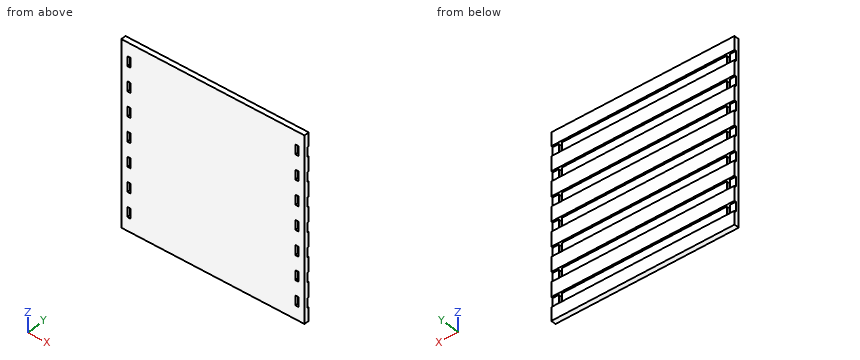
from build123d import *

# Parameters (mm, degrees)
SKETCH1_W           = 190.5
SKETCH1_H           = 190.5
BOSS_EXTRUDE1_DEPTH = 5.159375
SKETCH2_W           = 190.5
SKETCH2_H           = 10.16
CUT_EXTRUDE1_DEPTH  = 1.778
SKETCH3_W           = 3.175
SKETCH3_H           = 10.16
CUT_EXTRUDE3_DEPTH  = 4.381375
LPATTERN1_COUNT     = 7
LPATTERN1_PITCH     = 25.4


with BuildPart() as part:
    # Sketch1 → Boss-Extrude1 (new body)
    with BuildSketch(Plane(origin=(0, 0, 0), x_dir=(1, 0, 0), z_dir=(0, 1, 0))):
        Rectangle(SKETCH1_W, SKETCH1_H)
    extrude(amount=BOSS_EXTRUDE1_DEPTH)

    # Sketch2 → Cut-Extrude1 (cut)
    with BuildSketch(Plane(origin=(0, 5.159375, 0), x_dir=(1, 0, 0), z_dir=(0, 1, 0))):
        with Locations((0, 76.2)):
            Rectangle(SKETCH2_W, SKETCH2_H)
        with Locations((0, 50.8)):
            Rectangle(SKETCH2_W, SKETCH2_H)
        with Locations((0, 25.4)):
            Rectangle(SKETCH2_W, SKETCH2_H)
        Rectangle(SKETCH2_W, SKETCH2_H)
        with Locations((0, -25.4)):
            Rectangle(SKETCH2_W, SKETCH2_H)
        with Locations((0, -50.8)):
            Rectangle(SKETCH2_W, SKETCH2_H)
        with Locations((0, -76.2)):
            Rectangle(SKETCH2_W, SKETCH2_H)
    extrude(amount=-CUT_EXTRUDE1_DEPTH, mode=Mode.SUBTRACT)

    # Sketch3 → Cut-Extrude3 (cut, through all)
    with BuildSketch(Plane(origin=(0, 3.381375, 0), x_dir=(1, 0, 0), z_dir=(0, 1, 0))):
        with Locations((-87.3125, 76.2)):
            Rectangle(SKETCH3_W, SKETCH3_H)
        with Locations((87.3125, 76.2)):
            Rectangle(SKETCH3_W, SKETCH3_H)
    cut_extrude3 = extrude(amount=-CUT_EXTRUDE3_DEPTH, mode=Mode.SUBTRACT)

    # LPattern1: Cut-Extrude3 ×7
    with Locations(*[(0, 0, i * LPATTERN1_PITCH) for i in range(1, LPATTERN1_COUNT)]):
        add(cut_extrude3, mode=Mode.SUBTRACT)


solid = part.part
Input: part model. Units: mm. Frame: model coordinates. Give positions to 0.01 mm unless a question says otherwise; leave off trailing zeros. Order: outer loops, then holes, each group sorted by start corner. A loop starts at its lowest first (then second) coordinate and runs counter-clockwise, first axis right, second up.
Q1. Section B-B on y = 4.35. State how many separate pieces and enclosed holes the cut face has, and give its area (3 significant figures).
Checked values:
separate pieces: 8
enclosed holes: 0
area: 22,700 mm2
Q2. Contact query for a flat-ended pin moving along its axis: pin 1 Ø3 at (x, z) = (93, -48.5) entering from +Y. Output: stop coordinate, or through.
Checked values:
pin 1: stops at y = 3.38
Q3. Section A-A on z = -1. Output: boundary loops of the cut face in (x, y) (3 decimals), and give its area (3 significant figures).
Checked values:
outline: (-95.25, 0) - (-88.9, 0) - (-88.9, 3.381) - (-95.25, 3.381) - close; (-85.725, 0) - (85.725, 0) - (85.725, 3.381) - (-85.725, 3.381) - close; (88.9, 0) - (95.25, 0) - (95.25, 3.381) - (88.9, 3.381) - close
area: 623 mm2
Q4. Ray query, probe 1 along X at (y, z) = (2, -78) (3 decimals); probe 2 along Y at (x, z) = (-76, 81). Return the intervals inside material, ascending.
Checked values:
probe 1: x = -95.25 to -88.9, -85.725 to 85.725, 88.9 to 95.25
probe 2: y = 0 to 3.38
